Here's the drawing with two shaded views (mm, measured from the low corner). I have some questions. A direction names the side the tool comes from. Round coordinates to 2 decimals unless told otherwise and drop trailing zeros. Order: outer loops, then holes, each group sorted by start corner. A loop starts at its lowest first (then second) coordinate and runs counter-clockwise, first axis right, second up.
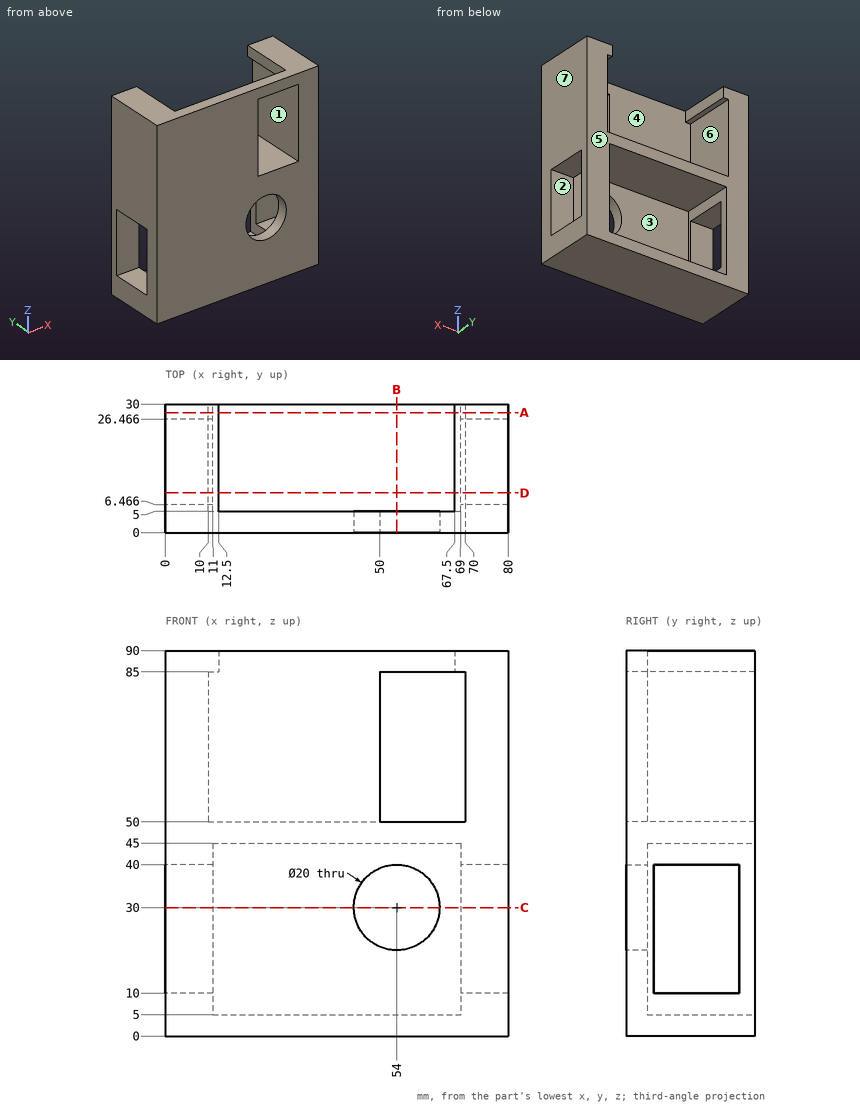
1. If we section it at B-B, the plane x = 54: Write out the boundary of the cut face in (y, z).
Evaluation:
outline: (0, 0) - (30, 0) - (30, 5) - (5, 5) - (5, 20) - (0, 20) - close; (0, 40) - (5, 40) - (5, 45) - (30, 45) - (30, 50) - (0, 50) - close; (0, 85) - (5, 85) - (5, 90) - (0, 90) - close
2. If we section it at D-D, the plane y = 9.25: Write out the boundary of the cut face in (x, z).
Evaluation:
outline: (0, 0) - (80, 0) - (80, 10) - (69, 10) - (69, 5) - (11, 5) - (11, 10) - (0, 10) - close; (0, 40) - (11, 40) - (11, 45) - (69, 45) - (69, 40) - (80, 40) - (80, 90) - (67.5, 90) - (67.5, 85) - (70, 85) - (70, 50) - (10, 50) - (10, 85) - (12.5, 85) - (12.5, 90) - (0, 90) - close
3. If we section it at C-C, the plane z = 30: Write out the boundary of the cut face in (x, y).
Evaluation:
outline: (0, 0) - (44, 0) - (44, 5) - (11, 5) - (11, 6.47) - (0, 6.47) - close; (0, 26.47) - (11, 26.47) - (11, 30) - (0, 30) - close; (64, 0) - (80, 0) - (80, 6.47) - (69, 6.47) - (69, 5) - (64, 5) - close; (69, 26.47) - (80, 26.47) - (80, 30) - (69, 30) - close
4. I'm going to push flat-ended pins straight in: P1, Ø2, axis at x = 35.5, y = 18, coming from the +Z side; P2, Ø12, axis at x = 44, z = 60.5, coming from the +Y side. Where does each tip first touch, or does it pass through?
Evaluation:
P1: stops at z = 50
P2: stops at y = 5
5. I need wall thicknesses on probe 1 along Z at (x, y) = (13.5, 25); probe 2 along X at (y, z) = (2.7, 30); probe 3 along Z at (x, y) = (68, 8.5). Which ranges of each line are inside material? Lowest first, please.
Evaluation:
probe 1: z = 0 to 5, 45 to 50
probe 2: x = 0 to 44, 64 to 80
probe 3: z = 0 to 5, 45 to 50, 85 to 90
6. If we mould it in two halves opening along X, with no side actions, what happens to the marked faces 4, 5, 6 and 7? For each: released by +X, released by -X, zero draft, split by the parting line, or undercut.
Evaluation:
face 4: undercut
face 5: zero draft
face 6: undercut
face 7: released by +X
7. On a 3-axis mill with a long thin cutter (end or side, diameter ignored), from which of +Z, -Z, +X, -X, +Y, -Y can I reach the whole of each face in a straight line? I mean the marked faces 1, 2 and 3. Say none if no direction works.
Evaluation:
face 1: +Y, -Y
face 2: +X, -X
face 3: +Y
8. If we section it at A-A, the plane y = 28: Write out the boundary of the cut face in (x, z).
Evaluation:
outline: (0, 0) - (80, 0) - (80, 90) - (67.5, 90) - (67.5, 85) - (70, 85) - (70, 50) - (10, 50) - (10, 85) - (12.5, 85) - (12.5, 90) - (0, 90) - close; hole (11, 5) - (69, 5) - (69, 45) - (11, 45) - close
